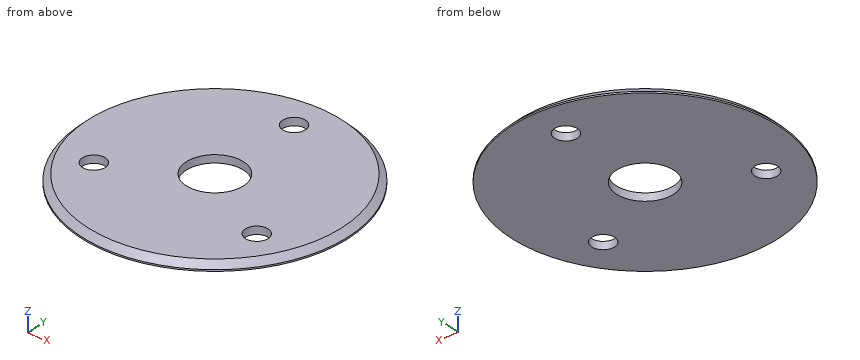
```python
from build123d import *

# Parameters (mm, degrees)
SKETCH1_R           = 35
SKETCH1_R_2         = 7.5
SKETCH1_R_3         = 3
BOSS_EXTRUDE1_DEPTH = 2
CHAMFER1_SIZE       = 1.6


with BuildPart() as part:
    # Sketch1 → Boss-Extrude1 (new body)
    with BuildSketch(Plane.XY):
        Circle(SKETCH1_R)
        Circle(SKETCH1_R_2, mode=Mode.SUBTRACT)
        with Locations((0, 25)):
            Circle(SKETCH1_R_3, mode=Mode.SUBTRACT)
        with Locations((21.650635095, -12.5)):
            Circle(SKETCH1_R_3, mode=Mode.SUBTRACT)
        with Locations((-21.650635095, -12.5)):
            Circle(SKETCH1_R_3, mode=Mode.SUBTRACT)
    extrude(amount=BOSS_EXTRUDE1_DEPTH)

    # Chamfer1
    chamfer1_edges = [part.edges().sort_by_distance(p)[0] for p in [
        (-35, 0, 2),
    ]]
    chamfer(chamfer1_edges, length=CHAMFER1_SIZE)


solid = part.part
```
Geometry check sheet. Reference: the model listing, model coordinates, mm. Give positions to 0.01 mm unless a question says otherwise; leave off trailing zeros. Order: outer loops, then holes, each group sorted by start corner. A loop starts at its lowest first (then second) coordinate and runs counter-clockwise, first axis right, second up. Notation, with made-up numbers: (50.5, 14) - (96.5, 14) arc R33 cw to (96.5, 44) - close; hole circle Ø5 at (29.25, 32). An arc over 180 degrees is marked (long way). Write item = value, one per line. Start each with the question number.
1) Section check A-A (y = 0). Enter the section's corners in (x, z).
2) Section check D-D (y = -12.5). Count the separate pieces of the cut face and the enclosed holes in it, then the cut area to 3 significant figures.
3) Section check B-B (x = 0). Enter the section's corners in (y, z).
4) Scan lines: L1, parallel to Y at x = 0, z = 0.65; L2, parallel to Y at x = 0, z = 1.45; L3, parallel to X at y = -11.5, z = 1.7. Record each from-to range of solid material in increasing order.
5) Section check C-C (z = 1.4). Enter the section's corners in (x, y), then the cut area to 3 significant figures.
Geometry check:
q1.outline = (-35, 0) - (-7.5, 0) - (-7.5, 2) - (-33.4, 2) - (-35, 0.4) - close; (7.5, 0) - (35, 0) - (35, 0.4) - (33.4, 2) - (7.5, 2) - close
q2.separate_pieces = 3
q2.enclosed_holes = 0
q2.area = 104 mm2
q3.outline = (-35, 0) - (-7.5, 0) - (-7.5, 2) - (-33.4, 2) - (-35, 0.4) - close; (7.5, 0) - (22, 0) - (22, 2) - (7.5, 2) - close; (28, 0) - (35, 0) - (35, 0.4) - (33.4, 2) - (28, 2) - close
q4.L1 = -34.75 to -7.5, 7.5 to 22, 28 to 34.75
q4.L2 = -33.95 to -7.5, 7.5 to 22, 28 to 33.95
q4.L3 = -31.68 to -24.48, -18.82 to 18.82, 24.48 to 31.68
q5.outline = circle Ø68 at (0, 0); hole circle Ø6 at (-21.65, -12.5); hole circle Ø15 at (0, 0); hole circle Ø6 at (0, 25); hole circle Ø6 at (21.65, -12.5)
q5.area = 3,370 mm2
